Input: part model. Units: mm. Frame: model coordinates. A direction names the side the tool comes from. Round coordinates to 2 decimals unless told otherwise and drop trailing zeros. Loops run counter-clockwise (first coordinate to the right, second up) from the corner with the lowest first, then second, coordinate; pieces in that order, holes last. Notation, with made-up numbers: (26, 24.5) - (35, 24.5) arc R16 cw to (35, 46.5) - close; hole circle Ø8 at (-17.75, 57). An arc over 180 degrees is marked (long way). One line per question, with ' | ' between items. Start each with the question number.
from build123d import *

# Parameters (mm, degrees)
F1_DEPTH = 25.4
F2_W     = 25.4
F2_H     = 25.4
F3_DEPTH = 25.4


with BuildPart() as f1:
    # F0 (on Front) → F1 (new body)
    with BuildSketch(Plane.XZ):
        with BuildLine():
            Line((-154.4574, 12.7), (-129.0574, 12.7))
            Line((-129.0574, 12.7), (-129.0574, -12.7))
            Line((-129.0574, -12.7), (-154.4574, -12.7))
            ThreePointArc((-154.4574, -12.7), (-136.437863, -22.141389), (-116.3574, -25.4))
            Line((-116.3574, -25.4), (0, -25.4))
            Line((0, -25.4), (116.3574, -25.4))
            ThreePointArc((116.3574, -25.4), (136.437863, -22.141389), (154.4574, -12.7))
            Line((154.4574, -12.7), (129.0574, -12.7))
            Line((129.0574, -12.7), (129.0574, 12.7))
            Line((129.0574, 12.7), (154.4574, 12.7))
            ThreePointArc((154.4574, 12.7), (143.298168, 39.640768), (116.3574, 50.8))
            Line((116.3574, 50.8), (0, 50.8))
            Line((0, 50.8), (-116.3574, 50.8))
            ThreePointArc((-116.3574, 50.8), (-143.298168, 39.640768), (-154.4574, 12.7))
        make_face()
        with BuildLine():
            ThreePointArc((-103.6574, 12.7), (-99.937656, 21.680256), (-90.9574, 25.4))
            Line((-90.9574, 25.4), (-38.1, 25.4))
            ThreePointArc((-38.1, 25.4), (-29.119744, 21.680256), (-25.4, 12.7))
            ThreePointArc((-25.4, 12.7), (-29.119744, 3.719744), (-38.1, 0))
            Line((-38.1, 0), (-90.9574, 0))
            ThreePointArc((-90.9574, 0), (-99.937656, 3.719744), (-103.6574, 12.7))
        make_face(mode=Mode.SUBTRACT)
        with BuildLine():
            Line((38.1, 25.4), (90.9574, 25.4))
            ThreePointArc((90.9574, 25.4), (99.937656, 21.680256), (103.6574, 12.7))
            ThreePointArc((103.6574, 12.7), (99.937656, 3.719744), (90.9574, 0))
            Line((90.9574, 0), (38.1, 0))
            ThreePointArc((38.1, 0), (29.119744, 3.719744), (25.4, 12.7))
            ThreePointArc((25.4, 12.7), (29.119744, 21.680256), (38.1, 25.4))
        make_face(mode=Mode.SUBTRACT)
    extrude(amount=F1_DEPTH)

    # F2 (on face) → F3 (cut)
    with BuildSketch(Plane.XZ.offset(25.4)):
        with Locations((0, 38.1)):
            Rectangle(F2_W, F2_H)
        with Locations((0, -12.7)):
            Rectangle(F2_W, F2_H)
    extrude(amount=-F3_DEPTH, mode=Mode.SUBTRACT)


solid = f1.part
(1) Pin query (flat end, axial travel): P1, Ø12.5, axis at x = 141.5, y = -12.5, coming from the +Z side; P2, Ø7.5, axis at y = -14.5, z = -2, coming from the -X side; P3, Ø7.5, axis at y = -18.5, z = -18, coming from the +X side. Return the tip coordinate at first contact, or that it passes through.
(2) Section D-D, the plane x = -6.5. Output: boundary loops of the cut face in (y, z).
(3) Pull-direction query (Z, two-part tool) for faces 5 (the face through (143.593, -12.522, 39.343)), 6 (the face through (-65, -13, 25.4)), 7 (the face through (-12.7, -13, -13)); classes: released by +Z, released by -Z, zero draft, split by the parting line, or undercut.
(4) Section C-C, the plane z = 36. Output: boundary loops of the cut face in (x, y).
(5) Line query: line 1 along Z through (x, y) = (-81, -11.5); line 2 along X through (y, z) = (-18, 1.5); line 3 along X through (y, z) = (-11.5, -1). Output: solid intervals per line, ascending. Write a range as from..to.
(6) Section A-A, the plane x = -44. Output: boundary loops of the cut face in (y, z).
(7) Reachability of faces 1 (the face through (129.057, -13, 0)), 2 (the face through (-142, -13, 12.7)), 3 (the face through (-64, -13, 0)), 4 (the face through (12.7, -13, 38)) from +Z, -Z, +X, -X, +Y, -Y: full face, straight path, thin tool, end or side. Return the list, or none.
(8) Section B-B, the plane y = -13.5. Output: boundary loops of the cut face in (x, z).
Derived:
1) P1: stops at z = 45.79 | P2: stops at x = -129.06 | P3: stops at x = 152.3
2) outline: (-25.4, 0) - (0, 0) - (0, 25.4) - (-25.4, 25.4) - close
3) face 5: released by +Z | face 6: undercut | face 7: zero draft
4) outline: (-146.5, -25.4) - (-12.7, -25.4) - (-12.7, 0) - (-146.5, 0) - close; (12.7, -25.4) - (146.5, -25.4) - (146.5, 0) - (12.7, 0) - close
5) line 1: z = -25.4..0, 25.4..50.8 | line 2: x = -129.06..-96.94, -32.11..32.11, 96.94..129.06 | line 3: x = -129.06..-12.7, 12.7..129.06
6) outline: (-25.4, -25.4) - (0, -25.4) - (0, 0) - (-25.4, 0) - close; (-25.4, 25.4) - (0, 25.4) - (0, 50.8) - (-25.4, 50.8) - close
7) face 1: +X, +Y, -Y | face 2: -X, +Y, -Y | face 3: +Y, -Y | face 4: +Z, +Y, -Y
8) outline: (-154.46, -12.7) arc R63.5 ccw to (-116.36, -25.4) - (-12.7, -25.4) - (-12.7, 0) - (12.7, 0) - (12.7, -25.4) - (116.36, -25.4) arc R63.5 ccw to (154.46, -12.7) - (129.06, -12.7) - (129.06, 12.7) - (154.46, 12.7) arc R38.1 ccw to (116.36, 50.8) - (12.7, 50.8) - (12.7, 25.4) - (-12.7, 25.4) - (-12.7, 50.8) - (-116.36, 50.8) arc R38.1 ccw to (-154.46, 12.7) - (-129.06, 12.7) - (-129.06, -12.7) - close; hole (-90.96, 0) - (-38.1, 0) arc R12.7 ccw to (-38.1, 25.4) - (-90.96, 25.4) arc R12.7 ccw to start; hole (38.1, 0) - (90.96, 0) arc R12.7 ccw to (90.96, 25.4) - (38.1, 25.4) arc R12.7 ccw to start
